```python
from build123d import *

# Parameters (mm, degrees)
SKETCH_1_W          = 45
SKETCH_1_H          = 45
EXTRUDE_1_DEPTH     = 2.5
EXTRUDE_2_DEPTH     = 50
SKETCH_3_R          = 5.5
CUT_EXTRUDE_1_DEPTH = 40.5
CUT_EXTRUDE_2_DEPTH = 40.5
SKETCH_5_W          = 5
SKETCH_5_H          = 39.075696326
EXTRUDE_3_DEPTH     = 10
CUT_EXTRUDE_3_DEPTH = 43.037848163
SKETCH_7_W          = 5.5
SKETCH_7_H          = 39.075696326
EXTRUDE_4_DEPTH     = 20
CUT_EXTRUDE_4_DEPTH = 46
CUT_EXTRUDE_5_DEPTH = 43.037848163


with BuildPart() as part:
    # 草图1 → 凸台-拉伸1 (new body)
    with BuildSketch(Plane.XY):
        with Locations((22.5, 22.5)):
            Rectangle(SKETCH_1_W, SKETCH_1_H)
    extrude(amount=EXTRUDE_1_DEPTH)

    # 草图2 → 凸台-拉伸2 (add)
    with BuildSketch(Plane.XY.offset(2.5)):
        Polygon((36.5, 22.5), (36.5, 0), (39.5, 0), (39.5, 45), (36.5, 45), align=None)
        Polygon((8.5, 45), (8.5, 22.5), (8.5, 0), (5.5, 0), (5.5, 45), align=None)
    extrude(amount=EXTRUDE_2_DEPTH)

    # 草图3 → 切除-拉伸1 (cut, through all)
    with BuildSketch(Plane(origin=(39.5, 0, 0), x_dir=(0, 0, -1), z_dir=(1, 0, 0))):
        with Locations((-42, 22.5)):
            Circle(SKETCH_3_R)
    extrude(amount=-CUT_EXTRUDE_1_DEPTH, mode=Mode.SUBTRACT)

    # 草图4 → 切除-拉伸2 (cut, through all)
    with BuildSketch(Plane(origin=(39.5, 0, 0), x_dir=(0, 0, -1), z_dir=(1, 0, 0))):
        with BuildLine():
            Line((-2.5, 45), (-2.5, 41.474247654))
            ThreePointArc((-2.5, 41.474247654), (-25.225749209, 40.564939101), (-46.358725725, 32.157571933))
            ThreePointArc((-46.358725725, 32.157571933), (-50.832231318, 28.283182945), (-52.5, 22.605006306))
            Line((-52.5, 22.605006306), (-52.5, 45))
            Line((-52.5, 45), (-2.5, 45))
        make_face()
        with BuildLine():
            Line((-52.5, 22.394993694), (-52.5, 0))
            Line((-52.5, 0), (-2.5, 0))
            Line((-2.5, 0), (-2.5, 3.525752346))
            ThreePointArc((-2.5, 3.525752346), (-25.225749209, 4.435060899), (-46.358725725, 12.842428067))
            ThreePointArc((-46.358725725, 12.842428067), (-50.832231318, 16.716817055), (-52.5, 22.394993694))
        make_face()
    extrude(amount=-CUT_EXTRUDE_2_DEPTH, mode=Mode.SUBTRACT)

    # 草图5 → 凸台-拉伸3 (add)
    with BuildSketch(Plane.XY.offset(2.5)):
        with Locations((11, 22.5)):
            Rectangle(SKETCH_5_W, SKETCH_5_H)
        with Locations((34, 22.5)):
            Rectangle(SKETCH_5_W, SKETCH_5_H)
    extrude(amount=EXTRUDE_3_DEPTH)

    # 草图6 → 切除-拉伸3 (cut, through all)
    with BuildSketch(Plane(origin=(0, 42.037848163, 0), x_dir=(1, 0, 0), z_dir=(0, 1, 0))):
        with BuildLine():
            Line((13.5, -2.5), (13.5, -12.5))
            Line((13.5, -12.5), (8.5, -12.5))
            ThreePointArc((8.5, -12.5), (9.861833326, -6.930916663), (13.5, -2.5))
        make_face()
        with BuildLine():
            Line((31.5, -2.5), (31.5, -12.5))
            Line((31.5, -12.5), (36.5, -12.5))
            ThreePointArc((36.5, -12.5), (35.138166674, -6.930916663), (31.5, -2.5))
        make_face()
    extrude(amount=-CUT_EXTRUDE_3_DEPTH, mode=Mode.SUBTRACT)

    # 草图7 → 凸台-拉伸4 (add)
    with BuildSketch(Plane.XY.offset(2.5)):
        with Locations((2.75, 22.5)):
            Rectangle(SKETCH_7_W, SKETCH_7_H)
        with Locations((42.25, 22.5)):
            Rectangle(SKETCH_7_W, SKETCH_7_H)
    extrude(amount=EXTRUDE_4_DEPTH)

    # 草图8 → 切除-拉伸4 (cut, through all)
    with BuildSketch(Plane(origin=(45, 0, 0), x_dir=(0, 0, -1), z_dir=(1, 0, 0))):
        with BuildLine():
            Line((-22.5, 41.085625399), (-22.5, 42.037848163))
            Line((-22.5, 42.037848163), (-17.008220021, 42.037848163))
            ThreePointArc((-17.008220021, 42.037848163), (-19.771631621, 41.662789638), (-22.5, 41.085625399))
        make_face()
        with BuildLine():
            Line((-22.5, 3.914374601), (-22.5, 2.962151837))
            Line((-22.5, 2.962151837), (-17.008220021, 2.962151837))
            ThreePointArc((-17.008220021, 2.962151837), (-19.771631621, 3.337210362), (-22.5, 3.914374601))
        make_face()
    extrude(amount=-CUT_EXTRUDE_4_DEPTH, mode=Mode.SUBTRACT)

    # 草图9 → 切除-拉伸5 (cut, through all)
    with BuildSketch(Plane(origin=(0, 2.962151837, 0), x_dir=(-1, 0, 0), z_dir=(0, -1, 0))):
        with BuildLine():
            Line((-39.5, -22.5), (-45, -22.5))
            Line((-45, -22.5), (-45, -2.5))
            ThreePointArc((-45, -2.5), (-41.339785895, -12.249691121), (-39.5, -22.5))
        make_face()
        with BuildLine():
            Line((-5.5, -22.5), (0, -22.5))
            Line((0, -22.5), (0, -2.5))
            ThreePointArc((0, -2.5), (-3.660214105, -12.249691121), (-5.5, -22.5))
        make_face()
    extrude(amount=-CUT_EXTRUDE_5_DEPTH, mode=Mode.SUBTRACT)


solid = part.part
```
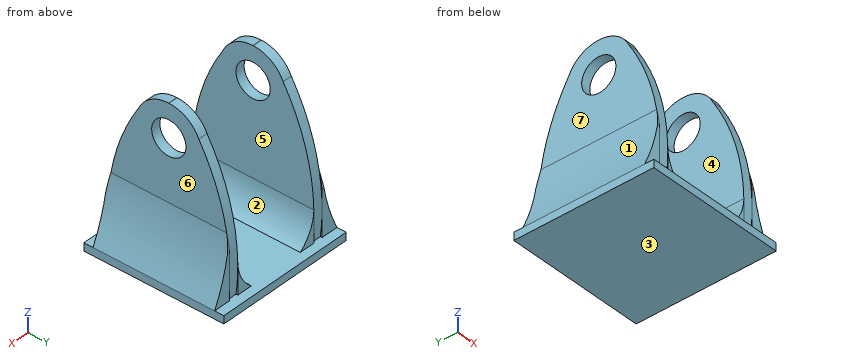
CAD build for the part. Positions are in the model's coordinates, mm. Face numbers are marked on the shaded views. A direction names the side the tool comes from. Round coordinates to 2 decimals unless told otherwise and drop trailing zeros. Write each loop counter-clockwise with the first axis right and the second up, starting at its lowest first coordinate (ties: lowest second). Pieces come first, ordered by that corner, then holes. Notation, with made-up numbers: (-33, 18.25) - (6, 18.25) arc R37 ccw to (6, 56.25) - close; hole circle Ø3 at (53.25, 0). An arc over 180 degrees is marked (long way). Return JSON: item names as keys, results as strings. Group by question number.
Item 1: Band-saw the part on C-C on z = 6.5. List the corners of the cut face in (x, y), plus the area to 3 significant figures.
Item 2: Band-saw the part on D-D on y = 10. List the corners of the cut face in (x, z), plus the area to 3 significant figures.
Item 3: 3-axis set-ups, long thin cutter, end or side, ignore diameter. For the marked faces 5, 6 and 7: which of +Z, -Z, +X, -X, +Y, -Y reach the whole face in a straight line?
Item 4: Band-saw the part on A-A on z = 42. List the corners of the cut face in (x, y), plus the area to 3 significant figures.
Item 5: Probe probe 1 along X at (y, z) = (17, 34); probe 2 along Z at (x, y) = (24.5, 4.5); probe 3 along Y at (x, z) = (7, 42). List the from-to ranges inside material, lowest first.
Item 6: Mould opens along X. For the marked faces 1, 2, 3 and 4 say: +X half, -X half, draft (parallel to the pull), parting line (faces both ways), or undercut.
Item 7: Flat gauge pins, fed straight in: pin 1 Ø6 at (x, z) = (43, 13) entering from -Y; pin 2 Ø2 at (y, z) = (12.5, 16) entering from +X; pin 3 Ø0.5 at (y, z) = (41.5, 8.5) entering from +X; pin 4 Ø1.5 at (x, z) = (12, 7.5) entering from +Y. Where does each tip first touch, or does it go through?
Item 8: Band-saw the part on B-B on y = 18. List the corners of the cut face in (x, z).
Resolved:
{
 "1": {"outline": "(1.75, 2.96) - (5.5, 2.96) - (5.5, 3.13) - (8.5, 3.13) - (8.5, 2.96) - (10.09, 2.96) - (10.09, 42.04) - (8.5, 42.04) - (8.5, 41.87) - (5.5, 41.87) - (5.5, 42.04) - (1.75, 42.04) - close; (34.91, 2.96) - (36.5, 2.96) - (36.5, 3.13) - (39.5, 3.13) - (39.5, 2.96) - (43.25, 2.96) - (43.25, 42.04) - (39.5, 42.04) - (39.5, 41.87) - (36.5, 41.87) - (36.5, 42.04) - (34.91, 42.04) - close", "area": "650 mm²"},
 "2": {"outline": "(0, 0) - (45, 0) - (45, 2.5) arc R57.44 cw to (39.5, 22.5) - (39.5, 41.21) - (36.5, 41.21) - (36.5, 12.5) arc R12.92 cw to (31.5, 2.5) - (13.5, 2.5) arc R12.92 cw to (8.5, 12.5) - (8.5, 41.21) - (5.5, 41.21) - (5.5, 22.5) arc R57.44 cw to (0, 2.5) - close", "area": "459 mm²"},
 "3": {"face 5": "+Z, +Y, -Y", "face 6": "+Z, +X, +Y, -Y", "face 7": "+Z, -X, +Y, -Y"},
 "4": {"outline": "(5.5, 10.4) - (8.5, 10.4) - (8.5, 17) - (5.5, 17) - close; (5.5, 28) - (8.5, 28) - (8.5, 34.6) - (5.5, 34.6) - close; (36.5, 10.4) - (39.5, 10.4) - (39.5, 17) - (36.5, 17) - close; (36.5, 28) - (39.5, 28) - (39.5, 34.6) - (36.5, 34.6) - close", "area": "79.2 mm²"},
 "5": {"probe 1": "x = 5.5 to 8.5, 36.5 to 39.5", "probe 2": "z = 0 to 2.5", "probe 3": "y = 10.4 to 17, 28 to 34.6"},
 "6": {"face 1": "-X half", "face 2": "undercut", "face 3": "draft", "face 4": "undercut"},
 "7": {"pin 1": "stops at y = 2.96", "pin 2": "stops at x = 40.66", "pin 3": "stops at x = 42.6", "pin 4": "passes through"},
 "8": {"outline": "(0, 0) - (45, 0) - (45, 2.5) arc R57.44 cw to (39.5, 22.5) - (39.5, 38.84) - (36.5, 38.84) - (36.5, 12.5) arc R12.92 cw to (31.5, 2.5) - (13.5, 2.5) arc R12.92 cw to (8.5, 12.5) - (8.5, 38.84) - (5.5, 38.84) - (5.5, 22.5) arc R57.44 cw to (0, 2.5) - close; (5.5, 45.16) - (8.5, 45.16) - (8.5, 51.54) - (5.5, 51.54) - close; (36.5, 45.16) - (39.5, 45.16) - (39.5, 51.54) - (36.5, 51.54) - close"}
}
